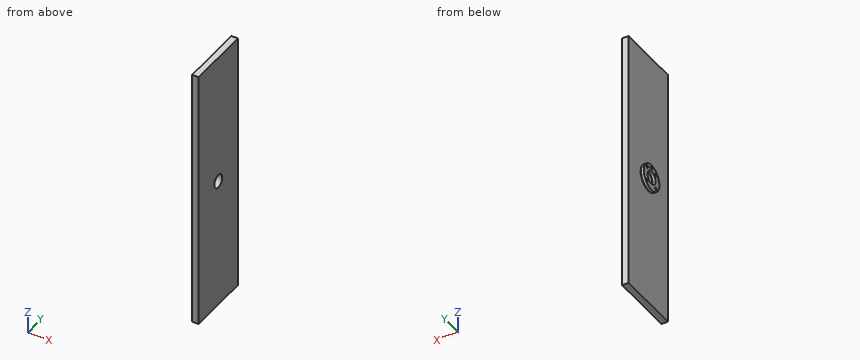
```python
from build123d import *

# Parameters (mm, degrees)
SKETCH1_W                      = 5
SKETCH1_H                      = 20
CUT_EXTRUDE1_REACH             = 2.2
SKETCH2_W                      = 2
SKETCH2_H                      = 1
F_20_0_20_DIAMETER_HOLE1_D     = 20
F_20_0_20_DIAMETER_HOLE1_DEPTH = 5
F_5_0_5_DIAMETER_HOLE1_D       = 5
F_5_0_5_DIAMETER_HOLE1_DEPTH   = 5
F_4_2_4_2_DIAMETER_HOLE1_D     = 4.2
F_4_2_4_2_DIAMETER_HOLE1_DEPTH = 5
CHAMFER1_SIZE                  = 0.5
CHAMFER1_SIZE2                 = 0.866025404
CHAMFER2_SIZE                  = 0.5
SKETCH9_W                      = 400
SKETCH9_H                      = 100
SKETCH9_R                      = 10
BOSS_EXTRUDE1_DEPTH            = 10


with BuildPart() as part:
    # Sketch1 → Revolve1 (revolve)
    with BuildSketch(Plane.XY.offset(889.1)):
        with Locations((530.5, 10)):
            Rectangle(SKETCH1_W, SKETCH1_H)
    revolve(axis=Axis((528, 0, 889.1), (1, 0, 0)))

    # Sketch2 → Cut-Extrude1 (cut, up to next)
    with BuildSketch(Plane(origin=(0, 0, 908.9), x_dir=(-1, 0, 0), z_dir=(0, 0, -1)), mode=Mode.PRIVATE) as cut_extrude1_sk1:
        with Locations((-529.5, 0)):
            Rectangle(SKETCH2_W, SKETCH2_H)
    cut_extrude1_tool1 = extrude(cut_extrude1_sk1.sketch, amount=-CUT_EXTRUDE1_REACH, mode=Mode.PRIVATE) & part.part
    add(cut_extrude1_tool1.solids().sort_by_distance((529.5, 0, 908.9))[0], mode=Mode.SUBTRACT)

    # Ø20.0 (20) Diameter Hole1
    with Locations(Plane(origin=(533, 0, 0), x_dir=(0, 0, -1), z_dir=(1, 0, 0))):
        with Locations((-889.1, 0)):
            Hole(F_20_0_20_DIAMETER_HOLE1_D / 2, depth=F_20_0_20_DIAMETER_HOLE1_DEPTH)

    # Ø5.0 (5) Diameter Hole1
    with Locations(Plane.ZY.offset(-528)):
        with Locations((904.85, 0)):
            Hole(F_5_0_5_DIAMETER_HOLE1_D / 2, depth=F_5_0_5_DIAMETER_HOLE1_DEPTH)

    # Ø4.2 (4.2) Diameter Hole1
    with Locations(Plane.ZY.offset(-528)):
        with Locations((900.236931804, 11.136931804), (877.963068196, -11.136931804), (877.963068196, 11.136931804), (900.236931804, -11.136931804)):
            Hole(F_4_2_4_2_DIAMETER_HOLE1_D / 2, depth=F_4_2_4_2_DIAMETER_HOLE1_DEPTH)

    # Chamfer1
    chamfer1_edges = [part.edges().sort_by_distance(p)[0] for p in [
        (533, -20, 889.1),
    ]]
    chamfer1_side = [part.faces().sort_by_distance(p)[0] for p in [
        (533, -19.434314575, 889.1),
    ]]
    chamfer(chamfer1_edges, length=CHAMFER1_SIZE, length2=CHAMFER1_SIZE2, reference=chamfer1_side[0])

    # Chamfer2
    chamfer2_edges = [part.edges().sort_by_distance(p)[0] for p in [
        (533, 0, 879.1),
    ]]
    chamfer(chamfer2_edges, length=CHAMFER2_SIZE)

    # Sketch9 → Boss-Extrude1 (add)
    with BuildSketch(Plane(origin=(533, 0, 0), x_dir=(0, 0, -1), z_dir=(1, 0, 0))):
        with Locations((-889.1, 0)):
            Rectangle(SKETCH9_W, SKETCH9_H)
        with Locations((-889.1, 0)):
            Circle(SKETCH9_R, mode=Mode.SUBTRACT)
    extrude(amount=BOSS_EXTRUDE1_DEPTH)


solid = part.part
```
Model file for the job. Use its own axes, mm. Give positions to 0.01 mm unless a question says otherwise; leave off trailing zeros. Loops run counter-clockwise (first coordinate to the right, second up) from the corner with the lowest first, then second, coordinate; pieces in that order, holes last. Notation, with made-up numbers: (6, 63) - (38, 63) arc R12 cw to (38, 86) - close; hole circle Ø10 at (68.5, 68). An arc over 180 degrees is marked (long way). One line per item, written item: value. Start each with the question number.
1. Probe L1, parallel to X at y = -37, z = 864; L2, parallel to Z at x = 536.25, y = -1.5; L3, parallel to Z at x = 530.5, y = -4. List the from-to ranges inside material, lowest first. Write a range as from..to.
2. Slice it at A-A (z = 889.1). List the corners of the cut face in (x, y), plus the area to 3 significant figures.
3. Pin check, flat tips, straight feed: pin 1 (12 mm diameter, centred on y = -21, z = 1007.5, fed in from -X); pin 2 (0.8 mm diameter, centred on x = 529.5, y = 0, fed in from +Z). Stop position of each tip, or through.
4. Slice it at B-B (z = 718.5). List the corners of the cut face in (x, y), plus the area to 3 significant figures.
Solution:
1. L1: x = 533..543
1. L2: z = 689.1..879.21, 898.99..1089.1
1. L3: z = 869.5..879.93, 898.27..908.7
2. outline: (528, -20) - (532.13, -20) - (533, -19.5) - (533, -50) - (543, -50) - (543, -10) - (533, -10) - (533, -10.5) - (532.5, -10) - (528, -10) - close; (528, 10) - (532.5, 10) - (533, 10.5) - (533, 10) - (543, 10) - (543, 50) - (533, 50) - (533, 19.5) - (532.13, 20) - (528, 20) - close
2. area: 899 mm^2
3. pin 1: stops at x = 533
3. pin 2: stops at z = 908.9
4. outline: (533, -50) - (543, -50) - (543, 50) - (533, 50) - close
4. area: 1,000 mm^2
